```python
from build123d import *

# Parameters (mm, degrees)
ESQUISSE1_W        = 200
ESQUISSE1_H        = 140
BOSS_EXTRU_1_DEPTH = 5
ESQUISSE3_R        = 2.5
BOSS_EXTRU_2_DEPTH = 20
ESQUISSE4_R        = 2.5
BOSS_EXTRU_3_DEPTH = 20
ESQUISSE6_R        = 2.5
BOSS_EXTRU_4_DEPTH = 20
ESQUISSE8_R        = 2.5
BOSS_EXTRU_5_DEPTH = 20


with BuildPart() as part:
    # Esquisse1 → Boss.-Extru.1 (new body)
    with BuildSketch(Plane(origin=(0, 0, 0), x_dir=(1, 0, 0), z_dir=(0, 1, 0))):
        Rectangle(ESQUISSE1_W, ESQUISSE1_H)
    extrude(amount=BOSS_EXTRU_1_DEPTH)

    # Esquisse3 → Boss.-Extru.2 (add)
    with BuildSketch(Plane.ZY.offset(100)):
        with Locations((67.5, 2.5)):
            Circle(ESQUISSE3_R)
    extrude(amount=BOSS_EXTRU_2_DEPTH)

    # Esquisse4 → Boss.-Extru.3 (add)
    with BuildSketch(Plane(origin=(100, 0, 0), x_dir=(0, 0, -1), z_dir=(1, 0, 0))):
        with Locations((-67.5, 2.5)):
            Circle(ESQUISSE4_R)
    extrude(amount=BOSS_EXTRU_3_DEPTH)

    # Esquisse6 → Boss.-Extru.4 (add)
    with BuildSketch(Plane.ZY.offset(100)):
        with Locations((-67.5, 2.5)):
            Circle(ESQUISSE6_R)
    extrude(amount=BOSS_EXTRU_4_DEPTH)

    # Esquisse8 → Boss.-Extru.5 (add)
    with BuildSketch(Plane(origin=(100, 0, 0), x_dir=(0, 0, -1), z_dir=(1, 0, 0))):
        with Locations((67.5, 2.5)):
            Circle(ESQUISSE8_R)
    extrude(amount=BOSS_EXTRU_5_DEPTH)


solid = part.part
```
Build history of the part. All positions in model axes, mm. A direction names the side the tool comes from. Give positions to 0.01 mm unless a question says otherwise; leave off trailing zeros. Loops run counter-clockwise (first coordinate to the right, second up) from the corner with the lowest first, then second, coordinate; pieces in that order, holes last.
1) Two-plate mould, pull along Z, no slides. Class faces 4 (the face through (-1, 2, -70)), 5 (the face through (-1, 5, -1)), 6 (the face through (100, 2, 1)): released by +Z, released by -Z, zero draft, split by the parting line, or undercut.
Values follow:
face 4: released by -Z
face 5: zero draft
face 6: undercut
2) Probe line 1 along X through (y, z) = (2.15, 57.5); line 2 along Z through (x, y) = (101, 3.4). List the from-to ranges inside material, lowest first.
Values follow:
line 1: x = -100 to 100
line 2: z = -69.83 to -65.17, 65.17 to 69.83
3) 3-axis set-ups, long thin cutter, end or side, ignore diameter. For faces 1 (the face through (-109.86, 3.251, 69.885)), 2 (the face through (-1, 0, -1)), 3 (the face through (109.86, 3.251, -69.885)): which of +Z, -Z, +X, -X, +Y, -Y reach the whole face in a straight line?
Values follow:
face 1: -X
face 2: +Z, -Z, +X, -X, -Y
face 3: +X
4) Band-saw the part on B-B on z = 53.5. List the corners of the cut face in (x, y).
Values follow:
outline: (-100, 0) - (100, 0) - (100, 5) - (-100, 5) - close
5) Drop flat-ended pins along their axis: P1, Ø5, axis at x = -1.5, z = 23, coming from the -Y side; P2, Ø2.5, axis at y = 2.5, z = 29, coming from the -X side. Give the stop position or say it passes through.
Values follow:
P1: stops at y = 0
P2: stops at x = -100
6) Band-saw the part on A-A on y = 1.6. List the corners of the cut face in (x, z), then the cut area to 3 significant figures.
Values follow:
outline: (-120, -69.83) - (-100, -69.83) - (-100, -70) - (100, -70) - (100, -69.83) - (120, -69.83) - (120, -65.17) - (100, -65.17) - (100, 65.17) - (120, 65.17) - (120, 69.83) - (100, 69.83) - (100, 70) - (-100, 70) - (-100, 69.83) - (-120, 69.83) - (-120, 65.17) - (-100, 65.17) - (-100, -65.17) - (-120, -65.17) - close
area: 28,400 mm2
